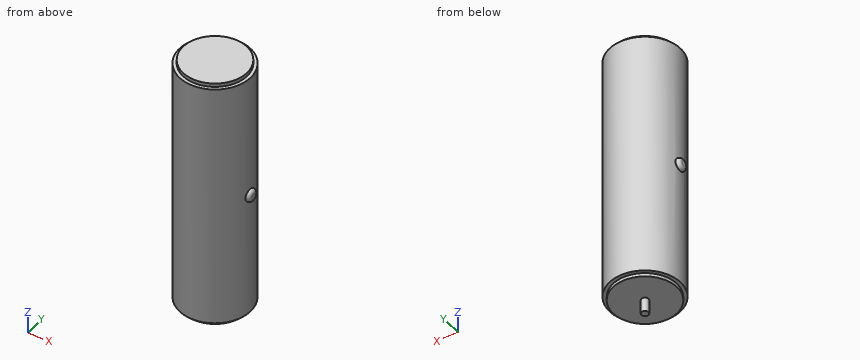
from build123d import *

# Parameters (mm, degrees)
SKETCH1_R                = 2.5
BOSS_EXTRUDE1_DEPTH      = 17.5
SKETCH2_R                = 2.25
BOSS_EXTRUDE2_DEPTH      = 0.25
BOSS_EXTRUDE3_START      = 0.25
SKETCH3_R                = 2.25
BOSS_EXTRUDE3_DEPTH      = 0.25
SKETCH4_R                = 0.25
BOSS_EXTRUDE4_DEPTH      = 1
BOSS_EXTRUDE5_DEPTH      = 2.75
BOSS_EXTRUDE5_DEPTH_BACK = 2.75
SKETCH5_R                = 0.442588638
FILLET1_R                = 0.25


with BuildPart() as part:
    # Sketch1 → Boss-Extrude1 (new body)
    with BuildSketch(Plane.XY):
        Circle(SKETCH1_R)
    extrude(amount=BOSS_EXTRUDE1_DEPTH)

    # Sketch2 → Boss-Extrude2 (add)
    with BuildSketch(Plane.XY.offset(17.5)):
        Circle(SKETCH2_R)
    extrude(amount=BOSS_EXTRUDE2_DEPTH)

    # Sketch3 → Boss-Extrude3 (add)
    with BuildSketch(Plane(origin=(0, 0, 0), x_dir=(-1, 0, 0), z_dir=(0, 0, -1)).offset(BOSS_EXTRUDE3_START)):
        with Locations(Location((0, 0, 0), (0, 0, 180))):
            Circle(SKETCH3_R)
    extrude(amount=-BOSS_EXTRUDE3_DEPTH)

    # Sketch4 → Boss-Extrude4 (add)
    with BuildSketch(Plane(origin=(0, 0, -0.25), x_dir=(-1, 0, 0), z_dir=(0, 0, -1))):
        Circle(SKETCH4_R)
    extrude(amount=BOSS_EXTRUDE4_DEPTH)

    # Sketch5 → Boss-Extrude5 (add, two sides: drawn at the far end of the back side and taken through both)
    with BuildSketch(Plane(origin=(0, 0, 0), x_dir=(0, 0, -1), z_dir=(1, 0, 0)).offset(-BOSS_EXTRUDE5_DEPTH_BACK)):
        with Locations((-8.75, 0)):
            Circle(SKETCH5_R)
    extrude(amount=BOSS_EXTRUDE5_DEPTH + BOSS_EXTRUDE5_DEPTH_BACK)

    # Fillet1
    fillet1_edges = [part.edges().sort_by_distance(p)[0] for p in [
        (-2.75, 0, 9.192588638),
        (2.75, 0, 9.192588638),
    ]]
    fillet(fillet1_edges, radius=FILLET1_R - 0.0001)  # a hair under: the kernel refuses the full size


solid = part.part
CAD build for the part. Positions are in the model's coordinates, mm. Round coordinates to 2 decimals unless told otherwise and drop trailing zeros. Write each loop counter-clockwise with the first axis right and the second up, starting at its lowest first coordinate (ties: lowest second). Pieces come first, ordered by that corner, then holes. Notation, with made-up numbers: (-5.5, -34) -> (18.5, -34) arc R19 ccw to (18.5, -11) -> close; hole circle Ø4 at (-8.75, -29.5). An arc over 180 degrees is marked (long way). Answer as a JSON object with one key per item and string values.
(1) Band-saw the part on D-D, the plane x = 1.55. List the corners of the cut face in (y, z), then the cut area to 3 significant figures.
Reported:
{"outline": "(-1.96, 0) -> (-1.63, 0) -> (-1.63, -0.25) -> (1.63, -0.25) -> (1.63, 0) -> (1.96, 0) -> (1.96, 17.5) -> (1.63, 17.5) -> (1.63, 17.75) -> (-1.63, 17.75) -> (-1.63, 17.5) -> (-1.96, 17.5) -> close", "area": "70.3 mm^2"}
(2) Probe probe 1 along Z at (x, y) = (1.75, 0.2); probe 2 along Y at (x, z) = (0.45, 1.25); probe 3 along X at (y, z) = (-0.9, 2.75). List the from-to ranges inside material, lowest first. Write a range as [from, to].
Reported:
{"probe 1": "z = [-0.25, 17.75]", "probe 2": "y = [-2.46, 2.46]", "probe 3": "x = [-2.33, 2.33]"}
(3) Band-saw the part on C-C, the plane y = -1.25. List the corners of the cut face in (x, z), then the cut area to 3 significant figures.
Reported:
{"outline": "(-2.17, 0) -> (-1.87, 0) -> (-1.87, -0.25) -> (1.87, -0.25) -> (1.87, 0) -> (2.17, 0) -> (2.17, 17.5) -> (1.87, 17.5) -> (1.87, 17.75) -> (-1.87, 17.75) -> (-1.87, 17.5) -> (-2.17, 17.5) -> close", "area": "77.6 mm^2"}
(4) Pin check, flat tips, straight feed: P1, Ø2, axis at y = 2, z = 14.5, coming from the -X side; P2, Ø3, axis at x = -0.5, z = 7.5, coming from the -Y side; P3, Ø1.5, axis at y = 0.5, z = 4.5, coming from the -X side. Stop position of each tip, or through.
Reported:
{"P1": "stops at x = -2.29", "P2": "stops at y = -2.5", "P3": "stops at x = -2.5"}
(5) Band-saw the part on B-B, the plane z = 2.75. List the corners of the cut face in (x, y), then the cut area to 3 significant figures.
Reported:
{"outline": "circle Ø5 at (0, 0)", "area": "19.6 mm^2"}
(6) Band-saw the part on A-A, the plane x = 0. List the corners of the cut face in (y, z), then the cut area to 4 significant figures.
Reported:
{"outline": "(-2.5, 0) -> (-2.25, 0) -> (-2.25, -0.25) -> (-0.25, -0.25) -> (-0.25, -1.25) -> (0.25, -1.25) -> (0.25, -0.25) -> (2.25, -0.25) -> (2.25, 0) -> (2.5, 0) -> (2.5, 17.5) -> (2.25, 17.5) -> (2.25, 17.75) -> (-2.25, 17.75) -> (-2.25, 17.5) -> (-2.5, 17.5) -> close", "area": "90.25 mm^2"}
